```python
from build123d import *

# Parameters (mm, degrees)
BOSS_EXTRUDE1_DEPTH = 3.175
SKETCH2_W           = 10
SKETCH2_H           = 3.175
SKETCH2_W_2         = 15
CUT_EXTRUDE1_DEPTH  = 4.1750001


with BuildPart() as part:
    # Sketch1 → Boss-Extrude1 (new body)
    with BuildSketch(Plane(origin=(0, 0, 0), x_dir=(1, 0, 0), z_dir=(0, 1, 0))):
        with BuildLine():
            add(Edge.make_bspline(
                [(0, 0), (3.07818129, 8.457233587), (19.262118608, 23.397882677), (40.36741362, 25), (42.5, 25)],
                knots=[0, 0, 0, 0, 0.479831935, 0.533146595, 0.533146595, 0.533146595, 0.533146595], degree=3))
            Line((0, 0), (42.5, 0))
            Line((42.5, 0), (42.5, 25))
        make_face()
        with BuildLine():
            Line((42.5, 25), (42.5, 0))
            Line((42.5, 0), (85, 0))
            add(Edge.make_bspline(
                [(42.5, 25), (44.36741362, 25), (63.21067639, 23.77153695), (81.92181871, 8.457233587), (85, 0)],
                knots=[0.533146595, 0.533146595, 0.533146595, 0.533146595, 0.579831935, 1, 1, 1, 1], degree=3))
        make_face()
    extrude(amount=BOSS_EXTRUDE1_DEPTH)

    # Sketch2 → Cut-Extrude1 (cut, through all)
    with BuildSketch(Plane.XZ):
        with Locations((68.175, -1.5875)):
            Rectangle(SKETCH2_W, SKETCH2_H)
        Polygon((60.762, 0), (60.762, -16), (63.175, -16), (63.175, -3.175), (63.175, 0), align=None)
        with Locations((42.5, -1.5875)):
            Rectangle(SKETCH2_W_2, SKETCH2_H)
        Polygon((24.238, -16), (24.238, 0), (21.825, 0), (21.825, -3.175), (21.825, -16), align=None)
        with Locations((16.825, -1.5875)):
            Rectangle(SKETCH2_W, SKETCH2_H)
    extrude(amount=-CUT_EXTRUDE1_DEPTH, mode=Mode.SUBTRACT)


solid = part.part
```
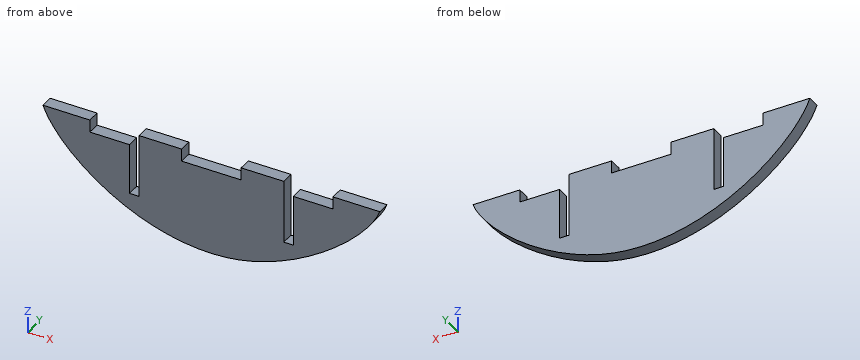
Check sheet for the modelled part. Datum: model origin and axes. Units: mm. Coordinates: 2 decimals unless noted, no trailing zeros. Use one line per item in the form item = value.
Item 1: Sectioned sample at A-A, the plane z = -13. State how many separate pieces and enclosed holes the cut face has, and give its area (3 significant figures).
Answer below:
separate_pieces = 3
enclosed_holes = 0
area = 186 mm^2
Item 2: Material ranges on L1, parallel to X at y = 2.65, z = -7.25 (3 decimals); L2, parallel to X at y = 1, z = -14.5 (3 decimals); L3, parallel to Z at x = 49.5, y = 3 (3 decimals), recorded low to high. Write a range as from..to.
Answer below:
L1 = 4.53..21.825, 24.238..60.762, 63.175..80.17
L2 = 12.357..21.825, 24.238..60.762, 63.175..71.891
L3 = -24.398..-3.175
Item 3: Gauge pin test, flat ends, axial feed: pin 1 Ø1 at (y, z) = (2.5, -1.5) entering from +X; pin 2 Ø1.9 at (x, y) = (62, 2) entering from +Z; pin 3 Ø1.6 at (y, z) = (2, -9.5) entering from +X. Record the tip position at first contact, or that the pin passes through.
Answer below:
pin_1 = 84.58
pin_2 = -16
pin_3 = 78.78
